from build123d import *

# Parameters (mm, degrees)
SKETCH1_W           = 457.2
SKETCH1_H           = 101.6
BASE_FLANGE1_DEPTH  = 12.7
SKETCH6_W           = 12.7
SKETCH6_H           = 292.1
BOSS_EXTRUDE1_DEPTH = 101.6
SKETCH9_W           = 12.7
SKETCH9_H           = 292.1
BOSS_EXTRUDE2_DEPTH = 101.6
CUT_EXTRUDE1_REACH  = 560.8
SKETCH12_R          = 14.985
FILLET1_R           = 50.8
FILLET2_R           = 50.8
CUT_EXTRUDE2_REACH  = 560.8
SKETCH13_R          = 14.985


# Sheet-metal steps are written as plain solids
with BuildPart() as part:
    # Sketch1 → Base-Flange1 (new body)
    with BuildSketch(Plane.XY):
        with Locations((228.6, 50.8)):
            Rectangle(SKETCH1_W, SKETCH1_H)
    extrude(amount=BASE_FLANGE1_DEPTH)

    # Sketch6 → Boss-Extrude1 (add, through all)
    with BuildSketch(Plane.XZ):
        with Locations((6.35, 158.75)):
            Rectangle(SKETCH6_W, SKETCH6_H)
    extrude(amount=-BOSS_EXTRUDE1_DEPTH)

    # Sketch9 → Boss-Extrude2 (add, through all)
    with BuildSketch(Plane.XZ):
        with Locations((450.85, 158.75)):
            Rectangle(SKETCH9_W, SKETCH9_H)
    extrude(amount=-BOSS_EXTRUDE2_DEPTH)

    # Sketch12 → Cut-Extrude1 (cut, up to next)
    with BuildSketch(Plane(origin=(457.2, 0, 0), x_dir=(0, 0, -1), z_dir=(1, 0, 0)), mode=Mode.PRIVATE) as cut_extrude1_sk1:
        with Locations((-246.361498901, 50.8)):
            Circle(SKETCH12_R)
    cut_extrude1_tool1 = extrude(cut_extrude1_sk1.sketch, amount=-CUT_EXTRUDE1_REACH, mode=Mode.PRIVATE) & part.part
    add(cut_extrude1_tool1.solids().sort_by_distance((457.2, 50.8, 246.361499))[0], mode=Mode.SUBTRACT)

    # Fillet1
    fillet1_edges = [part.edges().sort_by_distance(p)[0] for p in [
        (450.85, 0, 304.8),
        (450.85, 101.6, 304.8),
    ]]
    fillet(fillet1_edges, radius=FILLET1_R - 0.0001)  # a hair under: the kernel refuses the full size

    # Fillet2
    fillet2_edges = [part.edges().sort_by_distance(p)[0] for p in [
        (6.35, 0, 304.8),
        (6.35, 101.6, 304.8),
    ]]
    fillet(fillet2_edges, radius=FILLET2_R - 0.0001)  # a hair under: the kernel refuses the full size

    # Sketch13 → Cut-Extrude2 (cut, up to next)
    with BuildSketch(Plane.ZY, mode=Mode.PRIVATE) as cut_extrude2_sk1:
        with Locations(Location((76.2, 50.8, 0), (0, 0, 270))):
            Circle(SKETCH13_R)
    cut_extrude2_tool1 = extrude(cut_extrude2_sk1.sketch, amount=-CUT_EXTRUDE2_REACH, mode=Mode.PRIVATE) & part.part
    add(cut_extrude2_tool1.solids().sort_by_distance((0, 50.8, 76.2))[0], mode=Mode.SUBTRACT)


solid = part.part
Design review of the part built by this model. Coordinates are the model's own, in mm. A direction names the side the tool comes from. Give positions to 0.01 mm unless a question says otherwise; leave off trailing zeros. Write each loop counter-clockwise with the first axis right and the second up, starting at its lowest first coordinate (ties: lowest second). Pieces come first, ordered by that corner, then holes. Notation, with made-up numbers: M 22,-33.5 L 43,-33.5 A31 cw 43,-9.5 Z; hole C -31.5,52 d8. An arc over 180 degrees is marked long. Return JSON: item names as keys, results as strings. Group by question number.
Item 1: The part is to be moulded in two halves that separate along X. For faces 4 (the flat face through (12.7, 50, 157)), 5 (the flat face through (0, 50, 150)), 6 (the cylindrical face through (6.439, 14.486, 289.524)), say which applies: pulls with the +X half, pulls with the -X half, needs draft (parallel to the pull), parting line crosses it, or undercut.
Item 2: Take a section at C-C (y = 26.5). Give the boundary of the cut face in (x, z), plus the area to 3 significant figures.
Item 3: Take a section at B-B (z = 76.2). Give the boundary of the cut face in (x, y) (3 decimals).
Item 4: Clearance check with flat-ended pins moving along their axes: pin 1 Ø2 at (y, z) = (15, 203.5) entering from -X; pin 2 Ø1 at (x, y) = (398, 79.5) entering from +Z. State where each tip first meets the part, or that it passes through.
Item 5: Tool access review of faces 1 (the cylindrical face through (450.94, 55.3, 232.07)), 2 (the cylindrical face through (6.3, 43.9, 62.9)), 3 (the flat face through (444.5, 50, 157)): name each direction out of +Z, -Z, +X, -X, +Y, -Y from which nothing blocks a thin tool from reaching the whole face with its end or side.
Item 6: Take a section at D-D (x = 333). Give the boundary of the cut face in (y, z).
Item 7: Take a section at A-A (z = 189.5). Give the boundary of the cut face in (x, y), plus the area to 3 significant figures.
Item 8: Wall thickness on line 1 along X through (y, z) = (88.5, 17); line 2 along Z through (x, y) = (4, 50); line 3 along Z through (x, y) = (227.5, 93): over which ranges is each line inside the solid? List them lowest first.
Return value:
{
 "1": {"face 4": "undercut", "face 5": "pulls with the -X half", "face 6": "needs draft"},
 "2": {"outline": "M 0,0 L 457.2,0 L 457.2,298.61 L 444.5,298.61 L 444.5,12.7 L 12.7,12.7 L 12.7,298.61 L 0,298.61 Z", "area": "13,100 mm2"},
 "3": {"outline": "M 0,0 L 12.7,0 L 12.7,35.815 L 0,35.815 Z; M 0,65.785 L 12.7,65.785 L 12.7,101.6 L 0,101.6 Z; M 444.5,0 L 457.2,0 L 457.2,101.6 L 444.5,101.6 Z"},
 "4": {"pin 1": "stops at x = 0", "pin 2": "stops at z = 12.7"},
 "5": {"face 1": "+X", "face 2": "-X", "face 3": "+Z, +Y, -Y"},
 "6": {"outline": "M 0,0 L 101.6,0 L 101.6,12.7 L 0,12.7 Z"},
 "7": {"outline": "M 0,0 L 12.7,0 L 12.7,101.6 L 0,101.6 Z; M 444.5,0 L 457.2,0 L 457.2,101.6 L 444.5,101.6 Z", "area": "2,580 mm2"},
 "8": {"line 1": "x = 0 to 12.7, 444.5 to 457.2", "line 2": "z = 0 to 61.24, 91.16 to 304.79", "line 3": "z = 0 to 12.7"}
}
